Can you work these out from the drawing? Everything is in mm from the part's minimum corner. A direction names the side the tool comes from. Coordinates: 2 decimals unless noted, no trailing zeros. Loops run counter-clockwise (first coordinate to the right, second up) from the corner with the lowest first, then second, coordinate; pieces in that order, holes last. Notation, with made-up numbers: (42.25, 60.5) - (74.25, 60.5) arc R24 cw to (74.25, 74.5) - close; hole circle Ø10 at (12.5, 53.25). An arc over 180 degrees is marked (long way). Use CSV: the item, a comma, the result in double quotes.
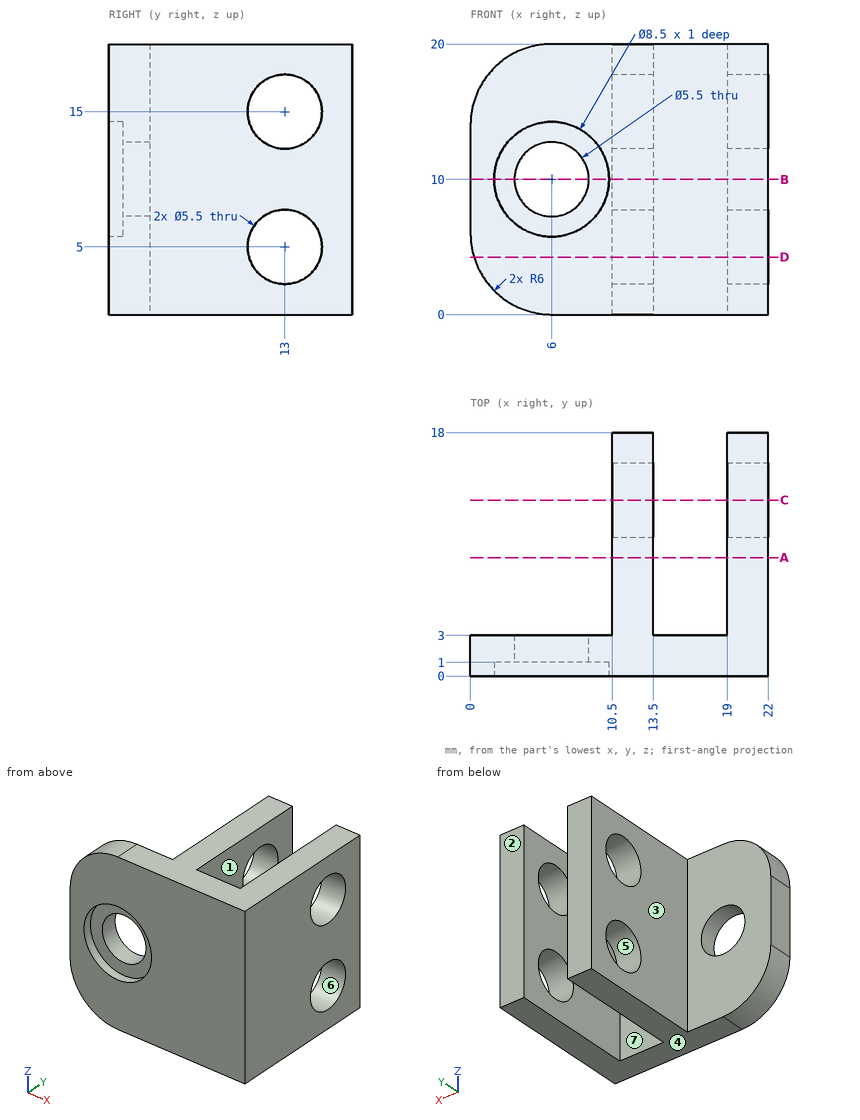
(1) Suppose I cut it at A-A (y = 8.75). Write out the boundary of the cut face in (x, z), plus the area to 3 significant figures.
Computed:
outline,"(10.5, 0) - (13.5, 0) - (13.5, 20) - (10.5, 20) - close; (19, 0) - (22, 0) - (22, 20) - (19, 20) - close"
area,"120 mm²"
(2) Suppose I cut it at C-C (y = 13). Write out the boundary of the cut face in (x, z), plus the area to 3 significant figures.
Computed:
outline,"(10.5, 0) - (13.5, 0) - (13.5, 2.25) - (10.5, 2.25) - close; (10.5, 7.75) - (13.5, 7.75) - (13.5, 12.25) - (10.5, 12.25) - close; (10.5, 17.75) - (13.5, 17.75) - (13.5, 20) - (10.5, 20) - close; (19, 0) - (22, 0) - (22, 2.25) - (19, 2.25) - close; (19, 7.75) - (22, 7.75) - (22, 12.25) - (19, 12.25) - close; (19, 17.75) - (22, 17.75) - (22, 20) - (19, 20) - close"
area,"54.0 mm²"
(3) Which directions (+Z, -Z, +X, -X, +Y, -Y) give clear straight access to the entire face, cutting with the end or side of a thin tool? Please do the marked faces 1, 2 and 3.
Computed:
face 1,"+Z, -Z, +Y"
face 2,"+Z, -Z, +X, -X, +Y"
face 3,"+Z, -Z, -X, +Y"
(4) Suppose I cut it at D-D (z = 4.25). Write out the boundary of the cut face in (x, y), plus the area to 3 significant figures.
Computed:
outline,"(0.26, 0) - (22, 0) - (22, 10.35) - (19, 10.35) - (19, 3) - (13.5, 3) - (13.5, 10.35) - (10.5, 10.35) - (10.5, 3) - (0.26, 3) - close; (10.5, 15.65) - (13.5, 15.65) - (13.5, 18) - (10.5, 18) - close; (19, 15.65) - (22, 15.65) - (22, 18) - (19, 18) - close"
area,"123 mm²"
(5) Please list where these lines run through material, in increasing order: line 1 (Z direction, x = 20.55, y = 13); line 2 (X direction, y = 8.25, z = 8.5); line 3 (Z direction, x = 19.25, y = 12.25).
Computed:
line 1,"z = 0 to 2.25, 7.75 to 12.25, 17.75 to 20"
line 2,"x = 10.5 to 13.5, 19 to 22"
line 3,"z = 0 to 2.35, 7.65 to 12.35, 17.65 to 20"
(6) Thinking about a two-plate mould opening in Z: for the marked faces 4, 5, 6 and 7, which applies, +Z half, -Z half, draft (parallel to the pull), parting line (faces both ways), or undercut?
Computed:
face 4,"-Z half"
face 5,"undercut"
face 6,"undercut"
face 7,"draft"
(7) Suppose I cut it at B-B (z = 10). Write out the boundary of the cut face in (x, y), plus the area to 4 significant figures.
Computed:
outline,"(0, 0) - (1.75, 0) - (1.75, 1) - (3.25, 1) - (3.25, 3) - (0, 3) - close; (8.75, 1) - (10.25, 1) - (10.25, 0) - (22, 0) - (22, 18) - (19, 18) - (19, 3) - (13.5, 3) - (13.5, 18) - (10.5, 18) - (10.5, 3) - (8.75, 3) - close"
area,"136.5 mm²"
(8) Will these pins go through, and if not, where does the flat tip stop? pin 1 (4 mm diameter, centred on x = 4.5, z = 9.5, fed in from -Y); pin 2 (10 mm diameter, centred on x = 2.5, z = 14.5, fed in from +Y); pin 3 (1.5 mm diameter, centred on x = 3, y = 5.5, fed in from -Z); pin 4 (6.5 mm diameter, centred on y = 13, z = 15, fed in from -X).
Computed:
pin 1,"stops at y = 1"
pin 2,"stops at y = 3"
pin 3,"passes through"
pin 4,"stops at x = 10.5"
